from build123d import *

# Parameters (mm, degrees)
SKETCH_1_R      = 13
SKETCH_1_R_2    = 10
EXTRUDE_1_DEPTH = 6
FILLET_1_R      = 0.8
FILLET_2_R      = 0.2


# Read off the part's stored shape, not the designer's step: 压凹5
with BuildPart() as part:
    # 草图1 → 凸台-拉伸1 (new body)
    with BuildSketch(Plane.XY):
        Circle(SKETCH_1_R)
        Circle(SKETCH_1_R_2, mode=Mode.SUBTRACT)
    extrude(amount=EXTRUDE_1_DEPTH)

    # 压凹5 outline → 压凹5 (revolve, cut)
    with BuildSketch(Plane.XZ):
        with BuildLine():
            Line((13, 1), (13, 5))
            ThreePointArc((13, 5), (12, 3), (13, 1))
        make_face()
    revolve(axis=Axis((0, 0, 0), (0, 0, 1)), mode=Mode.SUBTRACT)

    # 圆角1
    fillet_1_edges = [part.edges().sort_by_distance(p)[0] for p in [
        (-10, 0, 0),
        (-10, 0, 6),
    ]]
    fillet(fillet_1_edges, radius=FILLET_1_R)

    # 圆角2
    fillet_2_edges = [part.edges().sort_by_distance(p)[0] for p in [
        (-13, 0, 0),
        (-13, 0, 6),
    ]]
    fillet(fillet_2_edges, radius=FILLET_2_R)


solid = part.part
Can you work these out from the model? Positions are in its coordinate system, mm. Round coordinates to 2 decimals unless told otherwise and drop trailing zeros. Write each loop counter-clockwise with the first axis right and the second up, starting at its lowest first coordinate (ties: lowest second). Pieces come first, ordered by that corner, then holes. Notation, with made-up numbers: M -32,53.5 L 6,53.5 A13 cw 6,62.5 Z; hole C 0.25,17 d2. An arc over 180 degrees is marked long. Use a Markdown table: item, result.
Item 1: I want a section at D-D (z = 4). List the corners of the cut face in (x, y) for me, and give its area (3 significant figures).
Found:
| item | result |
|---|---|
| outline | C 0,0 d24.42; hole C 0,0 d20 |
| area | 154 mm2 |
Item 2: We'd pull the mould along Y, two halves only. Please class faces 1 (the face through (-10.316, -7.91, 0.594)), 2 (the face through (-2.17, -9.76, 2.97)), 3 (the face through (-5.7, -9.4, 6)): released by +Y, released by -Y, zero draft, split by the parting line, or undercut.
Found:
| item | result |
|---|---|
| face 1 | split by the parting line |
| face 2 | undercut |
| face 3 | zero draft |
Item 3: I want a section at C-C (z = 2.3). List the corners of the cut face in (x, y) for me, and give its area (3 significant figures).
Found:
| item | result |
|---|---|
| outline | C 0,0 d24.2; hole C 0,0 d20 |
| area | 146 mm2 |
Item 4: I want a section at A-A (y = 0). List the corners of the cut face in (x, z) for me, and give its area (3 significant figures).
Found:
| item | result |
|---|---|
| outline | M -13,0.2 A0.2 ccw -12.8,0 L -10.8,0 A0.8 ccw -10,0.8 L -10,5.2 A0.8 ccw -10.8,6 L -12.8,6 A0.2 ccw -13,5.8 L -13,5 A2.5 cw -13,1 Z; M 10,0.8 A0.8 ccw 10.8,0 L 12.8,0 A0.2 ccw 13,0.2 L 13,1 A2.5 cw 13,5 L 13,5.8 A0.2 ccw 12.8,6 L 10.8,6 A0.8 ccw 10,5.2 Z |
| area | 29.8 mm2 |
Item 5: For pin 1 Ø1.5 at (x, y) = (8, -5.5) entering from +Z; pin 2 Ø2 at (x, z) = (4.5, 2.5) entering from +Y, each with a flat end and sliding along its axis, tell me the tip position at first contact or that it passes through.
Found:
| item | result |
|---|---|
| pin 1 | stops at z = 5.92 |
| pin 2 | stops at y = 11.75 |
Item 6: If I drill on line 1 along X through (y, z) = (6.5, 4.1); line 2 along Y through (x, z) = (0, 2.6); line 3 along Y through (x, z) = (0, 4.1) (3 decimals), over which ranges is the centre line in solid material (lowest first)? Write a range as [from, to].
Found:
| item | result |
|---|---|
| line 1 | x = [-10.39, -7.6], [7.6, 10.39] |
| line 2 | y = [-12.03, -10], [10, 12.03] |
| line 3 | y = [-12.255, -10], [10, 12.255] |
